Model file for the job. Use its own axes, mm. Face numbers are marked on the shaded views. A direction names the side the tool comes from. Round coordinates to 2 decimals unless told otherwise and drop trailing zeros. Loops run counter-clockwise (first coordinate to the right, second up) from the corner with the lowest first, then second, coordinate; pieces in that order, holes last. Notation, with made-up numbers: (-35.75, 32) -> (-17.75, 32) arc R13 cw to (-17.75, 53) -> close; hole circle Ø4 at (41, 41). An arc over 180 degrees is marked (long way). Use a Markdown table: item, result. Add a question column.
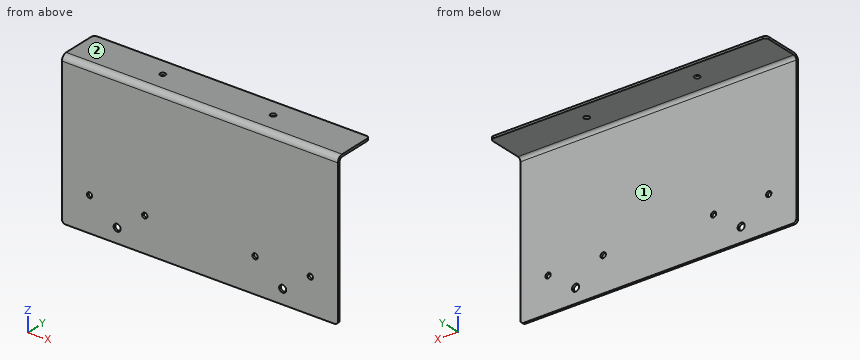
```python
from build123d import *

# Parameters (mm, degrees)
SKETCH1_W                    = 254
SKETCH1_H                    = 139.7
BASE_FLANGE1_DEPTH           = 2.052574
EDGE_FLANGE1_STRIP_W         = 14.210296
EDGE_FLANGE1_STRIP_H         = 2.052574
EDGE_FLANGE1_STRIP_CUT_DEPTH = 254
EDGE_FLANGE1_DEPTH           = 254
F_8_0_199_DIAMETER_HOLE1_D   = 5.0546
F_10_0_1935_DIAMETER_HOLE1_D = 4.9149
F_0_257_DIAMETER_HOLE1_D     = 6.5278
FILLET1_R                    = 3.175


# Sheet-metal steps are written as plain solids
with BuildPart() as part:
    # Sketch1 → Base-Flange1 (new body)
    with BuildSketch(Plane(origin=(0, 0, 0), x_dir=(1, 0, 0), z_dir=(0, 1, 0))):
        with Locations((127, 69.85)):
            Rectangle(SKETCH1_W, SKETCH1_H)
    extrude(amount=-BASE_FLANGE1_DEPTH)

    # Edge-Flange1 strip (across the edge) → Edge-Flange1 strip cut (cut)
    with BuildSketch(Plane(origin=(0, 0, 0), x_dir=(0, 0, -1), z_dir=(1, 0, 0))):
        with Locations((-2.052574, -1.026287)):
            Rectangle(EDGE_FLANGE1_STRIP_W, EDGE_FLANGE1_STRIP_H)
    extrude(amount=EDGE_FLANGE1_STRIP_CUT_DEPTH, mode=Mode.SUBTRACT)

    # Edge-Flange1 section (across the edge) → Edge-Flange1 (add)
    with BuildSketch(Plane(origin=(0, 0, 0), x_dir=(0, 0, -1), z_dir=(1, 0, 0))):
        with BuildLine():
            Line((0, 3), (0, 36.047426))
            Line((0, 36.047426), (2.052574, 36.047426))
            Line((2.052574, 36.047426), (2.052574, 3))
            ThreePointArc((2.052574, 3), (2.931253656, 0.878679656), (5.052574, 0))
            Line((5.052574, 0), (5.052574, -2.052574))
            ThreePointArc((5.052574, -2.052574), (1.479864662, -0.572709338), (0, 3))
        make_face()
    extrude(amount=EDGE_FLANGE1_DEPTH)

    # #8 (0.199) Diameter Hole1 (through all)
    with Locations(Plane(origin=(0, 0, -2.052574), x_dir=(-1, 0, 0), z_dir=(0, 0, -1))):
        with Locations((-177.8, 19.523713), (-76.2, 19.523713)):
            Hole(F_8_0_199_DIAMETER_HOLE1_D / 2)

    # #10 (0.1935) Diameter Hole1 (through all)
    with Locations(Plane(origin=(0, 0, 0), x_dir=(1, 0, 0), z_dir=(0, 1, 0))):
        with Locations((25.4, 107.95), (76.2, 107.95), (177.8, 107.95), (228.6, 107.95)):
            Hole(F_10_0_1935_DIAMETER_HOLE1_D / 2)

    # F (0.257) Diameter Hole1 (through all)
    with Locations(Plane(origin=(0, 0, 0), x_dir=(1, 0, 0), z_dir=(0, 1, 0))):
        with Locations((203.2, 126.48184), (50.8, 126.48184)):
            Hole(F_0_257_DIAMETER_HOLE1_D / 2)

    # Fillet1
    fillet1_edges = [part.edges().sort_by_distance(p)[0] for p in [
        (0, 36.047426, -1.026287),
        (254, 36.047426, -1.026287),
        (0, -1.026287, -139.7),
        (254, -1.026287, -139.7),
    ]]
    fillet(fillet1_edges, radius=FILLET1_R)


solid = part.part
```
1) Wall check: probe 1 along X at (y, z) = (-1, -107.95); probe 2 along Z at (x, y) = (50.8, -1.05); probe 3 along Y at (x, z) = (182, -91.5). Give the ranges that are in metal, low to high. Write a range as from..to.
2) Cut at B-B on z = -107.95. Write the cut outline in (x, y), and give its area (3 significant figures).
3) Cut at A-A on x = 228.6. Write the cut outline in (y, z), and give its area (3 significant figures).
4) Cut at D-D on x = 140.5. Write the cut outline in (y, z).
5) Cut at C-C on x = 76.2. Write the cut outline in (y, z).
6) Pin check, flat tips, straight feed: pin 1 Ø3 at (x, y) = (177.8, 19.52) entering from +Z; pin 2 Ø8 at (x, y) = (44.5, 19) entering from +Z; pin 3 Ø1.5 at (x, z) = (140.5, -54) entering from +Y; pin 4 Ø16.5 at (x, y) = (84.5, 26.5) entering from -Z. Stop position of each tip, or through.
7) Tool access for the marked faces 1 and 2: list every direction of +Z, -Z, +X, -X, +Y, -Y with a clear straight run to the whole face (end or side of a thin tool).
Established:
| question | item | result |
|---|---|---|
| 1 | probe 1 | x = 0..22.94, 27.86..73.74, 78.66..175.34, 180.26..226.14, 231.06..254 |
| 1 | probe 2 | z = -139.7..-129.75, -123.22..-2.03 |
| 1 | probe 3 | y = -2.05..0 |
| 2 | outline | (0, -2.05) -> (22.94, -2.05) -> (22.94, 0) -> (0, 0) -> close; (27.86, -2.05) -> (73.74, -2.05) -> (73.74, 0) -> (27.86, 0) -> close; (78.66, -2.05) -> (175.34, -2.05) -> (175.34, 0) -> (78.66, 0) -> close; (180.26, -2.05) -> (226.14, -2.05) -> (226.14, 0) -> (180.26, 0) -> close; (231.06, -2.05) -> (254, -2.05) -> (254, 0) -> (231.06, 0) -> close |
| 2 | area | 481 mm^2 |
| 3 | outline | (-2.05, -139.7) -> (0, -139.7) -> (0, -110.41) -> (-2.05, -110.41) -> close; (-2.05, -105.49) -> (0, -105.49) -> (0, -5.05) arc R3 cw to (3, -2.05) -> (36.05, -2.05) -> (36.05, 0) -> (3, 0) arc R5.05 ccw to (-2.05, -5.05) -> close |
| 3 | area | 347 mm^2 |
| 4 | outline | (-2.05, -139.7) -> (0, -139.7) -> (0, -5.05) arc R3 cw to (3, -2.05) -> (36.05, -2.05) -> (36.05, 0) -> (3, 0) arc R5.05 ccw to (-2.05, -5.05) -> close |
| 5 | outline | (-2.05, -139.7) -> (0, -139.7) -> (0, -110.41) -> (-2.05, -110.41) -> close; (-2.05, -105.49) -> (0, -105.49) -> (0, -5.05) arc R3 cw to (3, -2.05) -> (17, -2.05) -> (17, 0) -> (3, 0) arc R5.05 ccw to (-2.05, -5.05) -> close; (22.05, -2.05) -> (36.05, -2.05) -> (36.05, 0) -> (22.05, 0) -> close |
| 6 | pin 1 | passes through |
| 6 | pin 2 | stops at z = 0 |
| 6 | pin 3 | stops at y = 0 |
| 6 | pin 4 | stops at z = -2.05 |
| 7 | face 1 | -Z, +X, -X, +Y |
| 7 | face 2 | +Z, +X, -X, +Y, -Y |
